For this review, take the finished solid that the model builds, in its own axes (mm). Face numbers are marked on the shaded views. A direction names the side the tool comes from. Round coordinates to 2 decimals unless told otherwise and drop trailing zeros. Order: outer loops, then holes, each group sorted by start corner. A loop starts at its lowest first (then second) coordinate and runs counter-clockwise, first axis right, second up. Notation, with made-up numbers: (31.25, 21.5) -> (54.25, 21.5) arc R14 ccw to (54.25, 43.5) -> close; hole circle Ø3 at (26.5, -6.75). An arc over 180 degrees is marked (long way). Use a Markdown table: item, result. Add a question column.
1) Machinability: for the marked faces 1 and 2, which of the approach directions +Z, -Z, +X, -X, +Y, -Y give a long, thin tool a straight path to every point of the face, cutting with its end or side? Answer none if there is none.
2) Consider section B-B (z = -33.55). State the section outline as (x, y) points (3 decimals).
3) Clearance check with flat-ended pins moving along their axes: P1, Ø1.8, axis at x = -19.5, z = 28.5, coming from the +Y side; P2, Ø1, axis at x = -19.5, z = -30.5, coming from the +Y side. State where each tip first meets the part, or that it passes through.
4) Draft analysis for pull direction X (two halves, no side actions). For the marked faces 3, 4 and 5, state which applies: pulls with the +X half, pulls with the -X half, needs draft (parallel to the pull), parting line crosses it, or undercut.
5) Consider section C-C (y = 22). State the section outline as (x, z) points (3 decimals), plus the area to 3 significant figures.
6) Consider section A-A (x = 8.05). State the section outline as (y, z) points (3 decimals).
7) Consider section D-D (x = -10.5). State the section outline as (y, z) points (3 decimals), plus the area to 3 significant figures.
8) Wall thickness on line 1 along Z through (x, y) = (20.5, 33.5) (3 decimals); line 2 along X through (y, z) = (6, 10) (3 decimals); line 3 along Z through (x, y) = (13.5, 27.5) (3 decimals): over which ranges is each line inside the solid? List them lowest first. Write a range as [from, to].
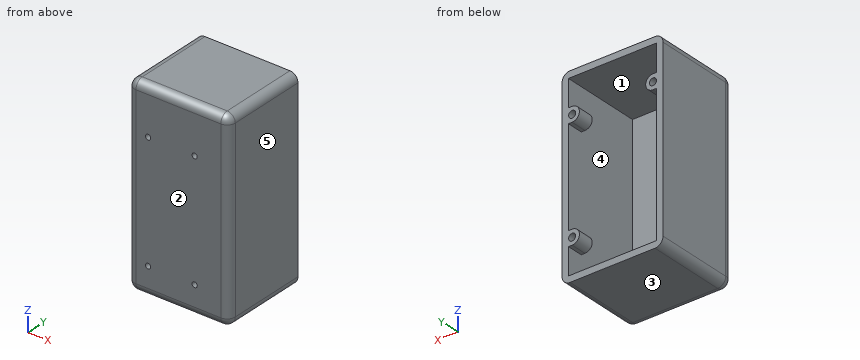
```python
from build123d import *

# Parameters (mm, degrees)
SKETCH1_W           = 50
SKETCH1_H           = 95.35
SKETCH1_W_2         = 43.65
SKETCH1_H_2         = 89
BOSS_EXTRUDE1_DEPTH = 40
SKETCH2_W           = 50
SKETCH2_H           = 95.35
BOSS_EXTRUDE2_DEPTH = 3.175
FILLET1_R           = 4
SKETCH3_R           = 1.3
CUT_EXTRUDE1_DEPTH  = 3.175
BOSS_EXTRUDE3_DEPTH = 8
SKETCH5_R           = 1.75
CUT_EXTRUDE2_DEPTH  = 5


with BuildPart() as part:
    # Sketch1 → Boss-Extrude1 (new body)
    with BuildSketch(Plane(origin=(0, 0, 0), x_dir=(1, 0, 0), z_dir=(0, 1, 0))):
        Rectangle(SKETCH1_W, SKETCH1_H)
        Rectangle(SKETCH1_W_2, SKETCH1_H_2, mode=Mode.SUBTRACT)
    extrude(amount=BOSS_EXTRUDE1_DEPTH)

    # Sketch2 → Boss-Extrude2 (add)
    with BuildSketch(Plane.XZ):
        Rectangle(SKETCH2_W, SKETCH2_H)
    extrude(amount=BOSS_EXTRUDE2_DEPTH)

    # Fillet1
    fillet1_edges = [part.edges().sort_by_distance(p)[0] for p in [
        (25, -3.175, 0),
        (0, -3.175, 47.675),
        (-25, -3.175, 0),
        (0, -3.175, -47.675),
        (25, 18.4125, 47.675),
        (-25, 18.4125, 47.675),
        (-25, 18.4125, -47.675),
        (25, 18.4125, -47.675),
    ]]
    fillet(fillet1_edges, radius=FILLET1_R)

    # Sketch3 → Cut-Extrude1 (cut)
    with BuildSketch(Plane(origin=(0, 0, 0), x_dir=(1, 0, 0), z_dir=(0, 1, 0))):
        with Locations(Location((-15, 33.55, 0), (0, 0, 270))):
            Circle(SKETCH3_R)
        with Locations(Location((8.05, 33.55, 0), (0, 0, 270))):
            Circle(SKETCH3_R)
        with Locations(Location((8.05, -24.5, 0), (0, 0, 270))):
            Circle(SKETCH3_R)
        with Locations(Location((-15, -24.5, 0), (0, 0, 270))):
            Circle(SKETCH3_R)
    extrude(amount=-CUT_EXTRUDE1_DEPTH, mode=Mode.SUBTRACT)

    # Sketch4 → Boss-Extrude3 (add)
    with BuildSketch(Plane(origin=(0, 40, 0), x_dir=(1, 0, 0), z_dir=(0, 1, 0))):
        with BuildLine():
            Line((-20, -24.075), (-21.825, -24.075))
            Line((-21.825, -24.075), (-21.825, -31.275))
            Line((-21.825, -31.275), (-20, -31.275))
            ThreePointArc((-20, -31.275), (-16.4, -27.675), (-20, -24.075))
        make_face()
        with BuildLine():
            Line((21.825, -31.275), (20, -31.275))
            ThreePointArc((20, -31.275), (16.4, -27.675), (20, -24.075))
            Line((20, -24.075), (21.825, -24.075))
            Line((21.825, -24.075), (21.825, -31.275))
        make_face()
        with BuildLine():
            Line((20, 24.075), (21.825, 24.075))
            Line((21.825, 24.075), (21.825, 31.275))
            Line((21.825, 31.275), (20, 31.275))
            ThreePointArc((20, 31.275), (16.4, 27.675), (20, 24.075))
        make_face()
    extrude(amount=-BOSS_EXTRUDE3_DEPTH)

    # Sketch5 → Cut-Extrude2 (cut)
    with BuildSketch(Plane(origin=(0, 40, 0), x_dir=(1, 0, 0), z_dir=(0, 1, 0))):
        with Locations(Location((-20, -27.675, 0), (0, 0, 270))):
            Circle(SKETCH5_R)
        with Locations(Location((20, -27.675, 0), (0, 0, 90))):
            Circle(SKETCH5_R)
        with Locations(Location((20, 27.675, 0), (0, 0, 270))):
            Circle(SKETCH5_R)
    extrude(amount=-CUT_EXTRUDE2_DEPTH, mode=Mode.SUBTRACT)


solid = part.part
```
Results list:
| question | item | result |
|---|---|---|
| 1 | face 1 | +Y |
| 1 | face 2 | +Z, -Z, +X, -X, -Y |
| 2 | outline | (-25, 0.825) arc R4 ccw to (-21, -3.175) -> (-16.3, -3.175) -> (-16.3, 0) -> (-21.825, 0) -> (-21.825, 40) -> (-25, 40) -> close; (-13.7, -3.175) -> (6.75, -3.175) -> (6.75, 0) -> (-13.7, 0) -> close; (9.35, -3.175) -> (21, -3.175) arc R4 ccw to (25, 0.825) -> (25, 40) -> (21.825, 40) -> (21.825, 0) -> (9.35, 0) -> close |
| 3 | P1 | y = 40 |
| 3 | P2 | y = 0 |
| 4 | face 3 | needs draft |
| 4 | face 4 | undercut |
| 4 | face 5 | pulls with the +X half |
| 5 | outline | (-25, -43.675) arc R4 ccw to (-21, -47.675) -> (21, -47.675) arc R4 ccw to (25, -43.675) -> (25, 43.675) arc R4 ccw to (21, 47.675) -> (-21, 47.675) arc R4 ccw to (-25, 43.675) -> close; hole (-21.825, -44.5) -> (21.825, -44.5) -> (21.825, 44.5) -> (-21.825, 44.5) -> close |
| 5 | area | 869 mm2 |
| 6 | outline | (-3.175, -43.675) arc R4 ccw to (0.825, -47.675) -> (40, -47.675) -> (40, -44.5) -> (0, -44.5) -> (0, -34.85) -> (-3.175, -34.85) -> close; (-3.175, -32.25) -> (0, -32.25) -> (0, 23.2) -> (-3.175, 23.2) -> close; (-3.175, 25.8) -> (0, 25.8) -> (0, 44.5) -> (40, 44.5) -> (40, 47.675) -> (0.825, 47.675) arc R4 ccw to (-3.175, 43.675) -> close |
| 7 | outline | (-3.175, -43.675) arc R4 ccw to (0.825, -47.675) -> (40, -47.675) -> (40, -44.5) -> (0, -44.5) -> (0, 44.5) -> (40, 44.5) -> (40, 47.675) -> (0.825, 47.675) arc R4 ccw to (-3.175, 43.675) -> close |
| 7 | area | 550 mm2 |
| 8 | line 1 | [-47.675, -44.5], [-31.275, -24.075], [24.075, 31.275], [44.5, 47.675] |
| 8 | line 2 | [-25, -21.825], [21.825, 25] |
| 8 | line 3 | [-47.675, -44.5], [44.5, 47.675] |
